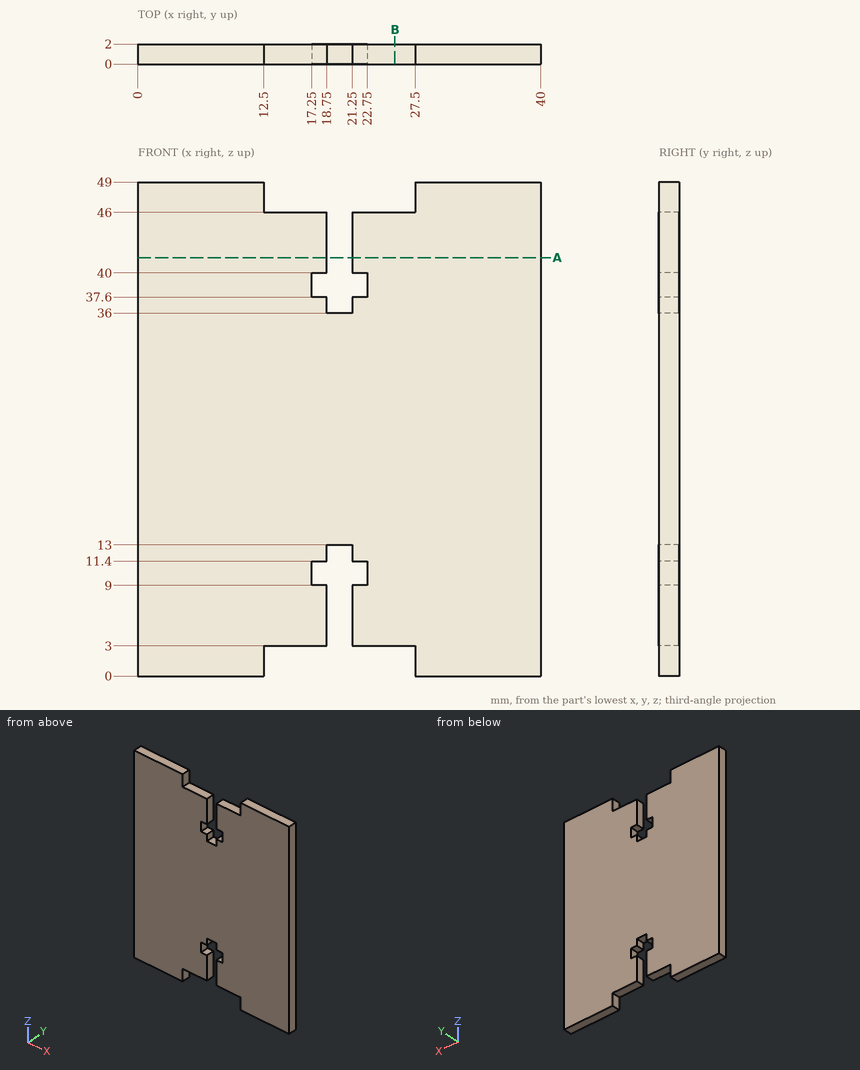
Job drawing, mm, ordinate dimensions from the low corner. One solid piece. Give positions to 0.01 mm unless a question says otherwise; leave off trailing zeros. Loops run counter-clockwise (first coordinate to the right, second up) from the corner with the lowest first, then second, coordinate; pieces in that order, holes last. Notation, with made-up numbers: (42.25, -7.75) -> (81.25, -7.75) arc R20 cw to (81.25, 27.25) -> close; hole circle Ø2 at (41, 24.25). An arc over 180 degrees is marked (long way). Write each question's results on one line, items separated by ' | '.
(1) Flat gauge pins, fed straight in: pin 1 Ø1.5 at (x, z) = (15, 18) entering from -Y; pin 2 Ø1 at (x, y) = (25, 1) entering from +Z. Where does each tip first touch, or does it go through?
Geometry results:
pin 1: stops at y = 0 | pin 2: stops at z = 46
(2) Probe line 1 along X through (y, z) = (1.5, 4); line 2 along Z through (x, y) = (20, 0.95); line 3 along X through (y, z) = (1.5, 47). List the from-to ranges inside material, lowest first.
Geometry results:
line 1: x = 0 to 18.75, 21.25 to 40 | line 2: z = 13 to 36 | line 3: x = 0 to 12.5, 27.5 to 40
(3) Cut at B-B on x = 25.5. List the corners of the cut face in (y, z).
Geometry results:
outline: (0, 3) -> (2, 3) -> (2, 46) -> (0, 46) -> close
(4) Cut at A-A on z = 41.5. List the corners of the cut face in (x, y).
Geometry results:
outline: (0, 0) -> (18.75, 0) -> (18.75, 2) -> (0, 2) -> close; (21.25, 0) -> (40, 0) -> (40, 2) -> (21.25, 2) -> close
